Build history of the part. All positions in model axes, mm. Face numbers are marked on the shaded views. A direction names the side the tool comes from. Coordinates: 2 decimals unless noted, no trailing zeros. Write each loop counter-clockwise with the first axis right and the second up, starting at its lowest first coordinate (ties: lowest second). Pieces come first, ordered by that corner, then holes.
```python
from build123d import *

# Parameters (mm, degrees)
CROQUIS1_W              = 75.25
CROQUIS1_H              = 80.25
CROQUIS1_W_2            = 60.4
CROQUIS1_H_2            = 60.4
SALIENTE_EXTRUIR1_DEPTH = 24
CROQUIS2_R              = 2.075
SALIENTE_EXTRUIR2_DEPTH = 7
CROQUIS3_R              = 1.5
SALIENTE_EXTRUIR3_DEPTH = 2
CROQUIS4_R              = 2.175
CROQUIS4_R_2            = 1.5
SALIENTE_EXTRUIR4_DEPTH = 20
CROQUIS5_W              = 4
CROQUIS5_H              = 5
CORTAR_EXTRUIR1_DEPTH   = 9.925
SALIENTE_EXTRUIR5_DEPTH = 2


with BuildPart() as part:
    # Croquis1 → Saliente-Extruir1 (new body)
    with BuildSketch(Plane.XY):
        with Locations((-58.191304348, -12.068115942)):
            Rectangle(CROQUIS1_W, CROQUIS1_H)
        with Locations((-58.191304348, -12.068115942)):
            Rectangle(CROQUIS1_W_2, CROQUIS1_H_2, mode=Mode.SUBTRACT)
    extrude(amount=SALIENTE_EXTRUIR1_DEPTH)

    # Croquis2 → Saliente-Extruir2 (add)
    with BuildSketch(Plane.XY.offset(24)):
        with Locations((-90.816304348, 23.056884058)):
            Circle(CROQUIS2_R)
        with Locations((-25.816304348, 23.056884058)):
            Circle(CROQUIS2_R)
        with Locations((-25.816304348, -46.943115942)):
            Circle(CROQUIS2_R)
        with Locations((-90.816304348, -46.943115942)):
            Circle(CROQUIS2_R)
    extrude(amount=SALIENTE_EXTRUIR2_DEPTH)

    # Croquis3 → Saliente-Extruir3 (add)
    with BuildSketch(Plane(origin=(0, 0, 0), x_dir=(-1, 0, 0), z_dir=(0, 0, -1))):
        Polygon((20.566304348, -19.843115942), (20.566304348, -52.193115942), (52.916304348, -52.193115942), align=None)
        with Locations((32.991304348, -36.868115942)):
            Circle(CROQUIS3_R, mode=Mode.SUBTRACT)
        Polygon((95.816304348, -4.293115942), (95.816304348, 28.056884058), (63.466304348, 28.056884058), align=None)
        with Locations((82.991304348, 13.131884058)):
            Circle(CROQUIS3_R, mode=Mode.SUBTRACT)
        Polygon((95.816304348, -19.843115942), (63.466304348, -52.193115942), (95.816304348, -52.193115942), align=None)
        with Locations((82.991304348, -36.868115942)):
            Circle(CROQUIS3_R, mode=Mode.SUBTRACT)
        Polygon((20.566304348, -4.293115942), (52.916304348, 28.056884058), (20.566304348, 28.056884058), align=None)
        with Locations((32.991304348, 13.131884058)):
            Circle(CROQUIS3_R, mode=Mode.SUBTRACT)
    extrude(amount=SALIENTE_EXTRUIR3_DEPTH)

    # Croquis4 → Saliente-Extruir4 (add)
    with BuildSketch(Plane.XY):
        with Locations((-82.991304348, 13.131884058)):
            Circle(CROQUIS4_R)
        with Locations((-82.991304348, 13.131884058)):
            Circle(CROQUIS4_R_2, mode=Mode.SUBTRACT)
        with Locations((-32.991304348, 13.131884058)):
            Circle(CROQUIS4_R)
        with Locations((-32.991304348, 13.131884058)):
            Circle(CROQUIS4_R_2, mode=Mode.SUBTRACT)
        with Locations((-32.991304348, -36.868115942)):
            Circle(CROQUIS4_R)
        with Locations((-32.991304348, -36.868115942)):
            Circle(CROQUIS4_R_2, mode=Mode.SUBTRACT)
        with Locations((-82.991304348, -36.868115942)):
            Circle(CROQUIS4_R)
        with Locations((-82.991304348, -36.868115942)):
            Circle(CROQUIS4_R_2, mode=Mode.SUBTRACT)
    extrude(amount=SALIENTE_EXTRUIR4_DEPTH)

    # Croquis5 → Cortar-Extruir1 (cut)
    with BuildSketch(Plane(origin=(0, -42.268115942, 0), x_dir=(1, 0, 0), z_dir=(0, 1, 0))):
        with Locations((-41.991304348, -21.5)):
            Rectangle(CROQUIS5_W, CROQUIS5_H)
    extrude(amount=-CORTAR_EXTRUIR1_DEPTH, mode=Mode.SUBTRACT)

    # Croquis6 → Saliente-Extruir5 (add)
    with BuildSketch(Plane(origin=(0, 0, 0), x_dir=(-1, 0, 0), z_dir=(0, 0, -1))):
        Polygon((42.991304348, 18.131884058), (52.916304348, 28.056884058), (63.466304348, 28.056884058), (73.391304348, 18.131884058), align=None)
        Polygon((27.991304348, 3.131884058), (27.991304348, -27.268115942), (20.566304348, -19.843115942), (20.566304348, -4.293115942), align=None)
        Polygon((42.991304348, -42.268115942), (52.916304348, -52.193115942), (63.466304348, -52.193115942), (73.391304348, -42.268115942), align=None)
        Polygon((88.391304348, -27.268115942), (88.391304348, 3.131884058), (95.816304348, -4.293115942), (95.816304348, -19.843115942), align=None)
    extrude(amount=SALIENTE_EXTRUIR5_DEPTH)


solid = part.part
```
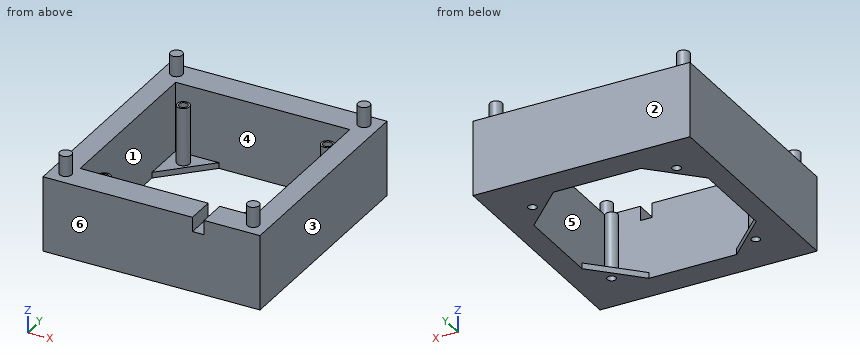
1. Probe line 1 along Y through (x, z) = (-74, 2); line 2 along X through (y, z) = (-33.5, 23); line 3 along Y through (x, z) = (-26, 28). List the from-to ranges inside material, lowest first.
Computed values:
line 1: y = -52.19 to -42.27, 18.13 to 28.06
line 2: x = -95.82 to -88.39, -27.99 to -20.57
line 3: y = -49.01 to -44.88, 20.99 to 25.12
2. Flat gauge pins, fed straight in: pin 1 (4 mm diameter, centred on x = -38.5, y = -39, fed in from +Z); pin 2 (5 mm diameter, centred on x = -82.99, y = 13.13, fed in from +Z). Where does each tip first touch, or does it go through?
Computed values:
pin 1: stops at z = 0
pin 2: stops at z = 20
3. 3-axis set-ups, long thin cutter, end or side, ignore diameter. For the marked faces 1 and 2: which of +Z, -Z, +X, -X, +Y, -Y reach the whole face in a straight line?
Computed values:
face 1: +Z
face 2: +Z, -Z, +X, -X, +Y
4. Saw through at C-C on x = -60. List the corners of the cut face in (y, z), plus the area to 3 significant figures.
Computed values:
outline: (-52.19, -2) - (-42.27, -2) - (-42.27, 24) - (-52.19, 24) - close; (18.13, -2) - (28.06, -2) - (28.06, 24) - (18.13, 24) - close
area: 516 mm2
5. Saw through at D-D on x = -39. List the corners of the cut face in (y, z), plus the area to 3 significant figures.
Computed values:
outline: (-52.19, -2) - (-38.28, -2) - (-38.28, 0) - (-42.27, 0) - (-42.27, 24) - (-52.19, 24) - close; (14.14, -2) - (28.06, -2) - (28.06, 24) - (18.13, 24) - (18.13, 0) - (14.14, 0) - close
area: 532 mm2
6. Mould opens along X. For the marked faces 3, 4, 5 and 6 say: +X half, -X half, draft (parallel to the pull), parting line (faces both ways), or undercut.
Computed values:
face 3: +X half
face 4: undercut
face 5: undercut
face 6: draft
7. Saw through at B-B on y = 0. List the corners of the cut face in (x, z).
Computed values:
outline: (-95.82, -2) - (-88.39, -2) - (-88.39, 24) - (-95.82, 24) - close; (-27.99, -2) - (-20.57, -2) - (-20.57, 24) - (-27.99, 24) - close
8. Saw through at A-A on z = 6.5. State how many separate pieces and enclosed holes the cut face has, plus the area to 3 significant figures.
Computed values:
separate pieces: 5
enclosed holes: 5
area: 2,420 mm2
